```python
from build123d import *

# Parameters (mm, degrees)
EXTRUDE_703_DEPTH          = 7.5
HOLE_WIZARD_M8_D           = 6.8
HOLE_WIZARD_M8_DEPTH       = 30
HOLE_WIZARD_M8_TIP         = 2.042926105
HOLE_WIZARD_M12_AT_2_COUNT = 2
HOLE_WIZARD_M12_AT_2_PITCH = 40
HOLE_WIZARD_M12_AT_3_COUNT = 2
HOLE_WIZARD_M12_AT_3_PITCH = 56.568542495
SKETCH_10_R                = 17
CUT_EXTRUDE_1_DEPTH        = 328.504072273
FK10_M4_D                  = 3.3
FK10_M4_CSINK_D            = 4.05
FK10_M4_CSINK_ANGLE        = 90


with BuildPart() as part:
    # Эскиз1 → Extrude 703 (new, symmetric)
    with BuildSketch(Plane(origin=(0, 0, 0), x_dir=(0, 0, -1), z_dir=(1, 0, 0))):
        Polygon((-80, 0), (0, 0), (80, 0), (80, 8), (200, 138.909090909), (200, 258.909090909), (150, 258.909090909), (-80, 8), align=None)
    extrude(amount=EXTRUDE_703_DEPTH, both=True)

    # Крепление к плите M8
    with Locations(Plane(origin=(0, 0, 0), x_dir=(-1, 0, 0), z_dir=(0, -1, 0))):
        with Locations((0, -50), (0, 50)):
            Hole(HOLE_WIZARD_M8_D / 2, depth=HOLE_WIZARD_M8_DEPTH)
            with Locations((0, 0, -(HOLE_WIZARD_M8_DEPTH + HOLE_WIZARD_M8_TIP / 2))):  # 118° drill point
                Cone(0, HOLE_WIZARD_M8_D / 2, HOLE_WIZARD_M8_TIP, mode=Mode.SUBTRACT)

    # Эскиз9 → К профилю M12 (revolve, cut)
    with BuildSketch(Plane(origin=(7.5, 196.809090909, -180), x_dir=(0, 0, -1), z_dir=(0, 1, 0))):
        Polygon((0, 0), (0, 15), (6.75, 15), (6.75, 6), (10, 6), (10, 0.025), (10.025, 0), align=None)
    hole_wizard_m12 = revolve(axis=Axis((13.85, 196.809090909, -180), (-1, 0, 0)), mode=Mode.SUBTRACT)

    # К профилю M12 at 2: К профилю M12 ×2
    with Locations(*[(0, -i * HOLE_WIZARD_M12_AT_2_PITCH, 0) for i in range(1, HOLE_WIZARD_M12_AT_2_COUNT)]):
        add(hole_wizard_m12, mode=Mode.SUBTRACT)

    # К профилю M12 at 3: К профилю M12 ×2
    with Locations(*[Vector(0, -0.7071067811865474, 0.7071067811865478) * (i * HOLE_WIZARD_M12_AT_3_PITCH) for i in range(1, HOLE_WIZARD_M12_AT_3_COUNT)]):
        add(hole_wizard_m12, mode=Mode.SUBTRACT)

    # Эскиз10 → Вырез-Вытянуть1 (cut, through all)
    with BuildSketch(Plane(origin=(7.5, 0, 0), x_dir=(0, 0, -1), z_dir=(1, 0, 0))):
        with Locations((140, 203.3)):
            Circle(SKETCH_10_R)
    extrude(amount=-CUT_EXTRUDE_1_DEPTH, mode=Mode.SUBTRACT)

    # FK10 - M4 (through all)
    with Locations(Plane(origin=(7.5, 0, 0), x_dir=(0, 0, -1), z_dir=(1, 0, 0))):
        with Locations((154.849242405, 218.149242405), (154.849242405, 188.450757595), (125.150757595, 188.450757595), (125.150757595, 218.149242405)):
            CounterSinkHole(FK10_M4_D / 2, FK10_M4_CSINK_D / 2, counter_sink_angle=FK10_M4_CSINK_ANGLE)


solid = part.part
```
Check sheet for the modelled part. Datum: model origin and axes. Units: mm. A direction names the side the tool comes from. Round coordinates to 2 decimals unless told otherwise and drop trailing zeros. Write each loop counter-clockwise with the first axis right and the second up, starting at its lowest first coordinate (ties: lowest second). Pieces come first, ordered by that corner, then holes. Notation, with made-up numbers: (30, 72) -> (36, 72) arc R26 cw to (36, 104) -> close; hole circle Ø9 at (44.5, 43.5). An arc over 180 degrees is marked (long way). Put each result on its own line as item: value.
(1) Sectioned sample at C-C (z = -0.5). Enter the section's corners in (x, y).
Values found:
outline: (-7.5, 0) -> (7.5, 0) -> (7.5, 95.82) -> (-7.5, 95.82) -> close
(2) Material ranges on line 1 (Y direction, x = 6.05, z = -140); line 2 (Z direction, x = 0, y = 10.75); line 3 (Y direction, x = 0.25, z = -145.5), recorded low to high.
Values found:
line 1: y = 73.45 to 146.81, 166.81 to 186.3, 220.3 to 248
line 2: z = -82.52 to -53.4, -46.6 to 46.6, 53.4 to 77.48
line 3: y = 79.45 to 152.9, 160.72 to 187.21, 219.39 to 254
(3) Mould release check, pull along Y, two halves, no side actions. Record for faces 1 (the face through (0.128, 31.688, 50.576)), 2 (the face through (-0.44, 15.21, 46.63)), 3 (the face through (4.53, 156.37, -130.01)): released by +Y, released by -Y, zero draft, split by the parting line, or undercut.
Values found:
face 1: released by -Y
face 2: zero draft
face 3: undercut
(4) Tool access check on faces 4 (the face through (1.5, 159, -173)), 5 (the face through (-0.44, 15.21, -53.37)), 6 (the face through (-2.9, 151.1, -183.6)). Record the directions out of +Z, -Z, +X, -X, +Y, -Y that give a thin tool (end or side, any length) a straight path to the whole face; none if there is none.
Values found:
face 4: +X
face 5: -Y
face 6: +X, -X
(5) Go/stop test with flat-tipped pins: pin 1 Ø2 at (y, z) = (218.15, -154.85) entering from -X (1 decimal); pin 2 Ø10 at (y, z) = (153.5, -138.5) entering from +X; pin 3 Ø1.5 at (x, z) = (-3, -149.5) entering from +Y; pin 4 Ø6 at (x, z) = (0, -50) entering from +Y. Record where each tip stops, or that it passes through.
Values found:
pin 1: passes through
pin 2: stops at x = 1.5
pin 3: stops at y = 258.91
pin 4: stops at y = 153.09
(6) Sectioned sample at D-D (y = 65.5). Enter the section's corners in (x, z), plus the area to 3 significant figures.
Values found:
outline: (-7.5, -132.71) -> (7.5, -132.71) -> (7.5, 27.29) -> (-7.5, 27.29) -> close
area: 2,400 mm^2
(7) Sectioned sample at A-A (z = -140). Enter the section's corners in (x, y) (3 decimals), plus the area to 3 significant figures.
Values found:
outline: (-7.5, 73.455) -> (7.5, 73.455) -> (7.5, 146.784) -> (7.475, 146.809) -> (1.5, 146.809) -> (1.5, 150.059) -> (-7.5, 150.059) -> close; (-7.5, 163.559) -> (1.5, 163.559) -> (1.5, 166.809) -> (7.475, 166.809) -> (7.5, 166.834) -> (7.5, 186.3) -> (-7.5, 186.3) -> close; (-7.5, 220.3) -> (7.5, 220.3) -> (7.5, 248) -> (-7.5, 248) -> close
area: 1,870 mm^2
(8) Sectioned sample at B-B (z = -180). Enter the section's corners in (x, y) (3 decimals), plus the area to 3 significant figures.
Values found:
outline: (-7.5, 117.091) -> (7.5, 117.091) -> (7.5, 146.784) -> (7.475, 146.809) -> (1.5, 146.809) -> (1.5, 150.059) -> (-7.5, 150.059) -> close; (-7.5, 163.559) -> (1.5, 163.559) -> (1.5, 166.809) -> (7.475, 166.809) -> (7.5, 166.834) -> (7.5, 186.784) -> (7.475, 186.809) -> (1.5, 186.809) -> (1.5, 190.059) -> (-7.5, 190.059) -> close; (-7.5, 203.559) -> (1.5, 203.559) -> (1.5, 206.809) -> (7.475, 206.809) -> (7.5, 206.834) -> (7.5, 258.909) -> (-7.5, 258.909) -> close
area: 1,640 mm^2
